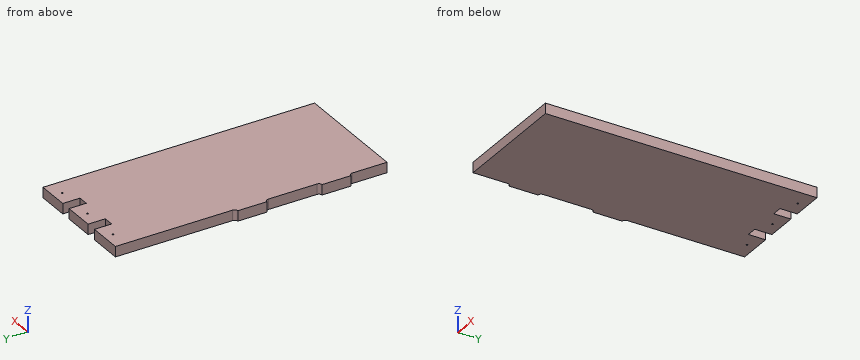
```python
from build123d import *

# Parameters (mm, degrees)
ESQUISSE1_R             = 0.127
ESQUISSE1_R_2           = 0.3999992
ESQUISSE1_R_3           = 0.4953
BOSS_EXTRU_1_DEPTH      = 1.55632912
ESQUISSE2_W             = 12.774737624
ESQUISSE2_H             = 41
ENL_V_MAT_EXTRU_1_DEPTH = 52.423945398


with BuildPart() as part:
    # Esquisse1 → Boss.-Extru.1 (new body)
    with BuildSketch(Plane(origin=(0, 0, 0), x_dir=(-1, 0, 0), z_dir=(0, 0, -1))):
        with BuildLine():
            Line((-12.23900032, 5.25), (-12.23900032, 0))
            Line((-12.23900032, 0), (0, 0))
            Line((0, 0), (0, 41))
            Line((0, 41), (-12.23900032, 41))
            Line((-12.23900032, 41), (-12.23900032, 23.299999237))
            ThreePointArc((-12.23900032, 23.299999237), (-12.74450016, 22.794499397), (-13.25, 23.299999237))
            Line((-13.25, 23.299999237), (-13.25, 41))
            Line((-13.25, 41), (-18.3939991, 41))
            Line((-18.3939991, 41), (-18.3939991, 38.400001526))
            Line((-18.3939991, 38.400001526), (-19.950000763, 38.400001526))
            Line((-19.950000763, 38.400001526), (-19.950000763, 41))
            Line((-19.950000763, 41), (-24.607000351, 41))
            Line((-24.607000351, 41), (-24.607000351, 38.400001526))
            Line((-24.607000351, 38.400001526), (-26.149999619, 38.400001526))
            Line((-26.149999619, 38.400001526), (-26.149999619, 41))
            Line((-26.149999619, 41), (-31, 41))
            Line((-31, 41), (-31, 0))
            Line((-31, 0), (-13.25, 0))
            Line((-13.25, 0), (-13.25, 5.25))
            ThreePointArc((-13.25, 5.25), (-12.74450016, 5.756000289), (-12.23900032, 5.25))
        make_face()
        with Locations(Location((-22.24999868, 39.64999944, 0), (0, 0, 180))):
            Circle(ESQUISSE1_R, mode=Mode.SUBTRACT)
        with Locations(Location((-28.44999898, 39.64999944, 0), (0, 0, 180))):
            Circle(ESQUISSE1_R, mode=Mode.SUBTRACT)
        with Locations(Location((-16.04999838, 39.64999944, 0), (0, 0, 180))):
            Circle(ESQUISSE1_R, mode=Mode.SUBTRACT)
        with Locations(Location((-8.7900002, 35.81500076, 0), (0, 0, 180))):
            Circle(ESQUISSE1_R_2, mode=Mode.SUBTRACT)
        with Locations(Location((-6.2500002, 38.35500076, 0), (0, 0, 180))):
            Circle(ESQUISSE1_R_2, mode=Mode.SUBTRACT)
        with Locations(Location((-3.7100002, 35.81500076, 0), (0, 0, 180))):
            Circle(ESQUISSE1_R_2, mode=Mode.SUBTRACT)
        with Locations(Location((-3.59000044, 6.14000042, 0), (0, 0, 180))):
            Circle(ESQUISSE1_R_3, mode=Mode.SUBTRACT)
        with Locations(Location((-1.05000044, 6.14000042, 0), (0, 0, 180))):
            Circle(ESQUISSE1_R_3, mode=Mode.SUBTRACT)
        with Locations(Location((-1.05000044, 1.06000042, 0), (0, 0, 180))):
            Circle(ESQUISSE1_R_3, mode=Mode.SUBTRACT)
        with Locations(Location((-1.05000044, 3.60000042, 0), (0, 0, 180))):
            Circle(ESQUISSE1_R_3, mode=Mode.SUBTRACT)
        with BuildLine():
            Line((-12.250000009, 17.899931304), (-12.251000404, 10.578000069))
            ThreePointArc((-12.251000404, 10.578000069), (-12.761750957, 10.078121146), (-13.25, 10.600000381))
            Line((-13.25, 10.600000381), (-13.25, 17.899999619))
            ThreePointArc((-13.25, 17.899999619), (-12.749965845, 18.399999615), (-12.250000009, 17.899931304))
        make_face(mode=Mode.SUBTRACT)
    extrude(amount=-BOSS_EXTRU_1_DEPTH)

    # Esquisse2 → Enlèv. mat.-Extru.1 (cut, through all)
    with BuildSketch(Plane.XY.offset(1.55632912)):
        with Locations((6.387368812, 20.5)):
            Rectangle(ESQUISSE2_W, ESQUISSE2_H)
    extrude(amount=-ENL_V_MAT_EXTRU_1_DEPTH, mode=Mode.SUBTRACT)


solid = part.part
```
Could you check a few things on this model? Use its own coordinates, in mm. Round coordinates to 2 decimals unless told otherwise and drop trailing zeros. Loops run counter-clockwise (first coordinate to the right, second up) from the corner with the lowest first, then second, coordinate; pieces in that order, holes last. Notation, with made-up numbers: (42.25, -12.75) - (92.25, -12.75) arc R27 cw to (92.25, 23.25) - close; hole circle Ø2 at (13.25, -24). An arc over 180 degrees is marked (long way). Answer as CSV lines item,"result".
1. For pin 1 Ø0.8 at (y, z) = (40, 1) entering from -X; pin 2 Ø0.5 at (x, z) = (25, 0.5) entering from +Y, each with a flat end and sliding along its axis, tell me the tip position at first contact or that it passes through.
Filled in:
pin 1,"stops at x = 13.25"
pin 2,"stops at y = 38.4"
2. Please list where these lines run through material, in increasing order: line 1 along X through (y, z) = (39.65, 1); line 2 along Y through (x, z) = (28.5, 1.1); line 3 along Y through (x, z) = (25.25, 0.3). Write a range as [from, to].
Filled in:
line 1,"x = [13.25, 15.92], [16.18, 18.39], [19.95, 22.12], [22.38, 24.61], [26.15, 28.32], [28.58, 31]"
line 2,"y = [0, 39.53], [39.77, 41]"
line 3,"y = [0, 38.4]"
3. I want a section at B-B on y = 14. List the corners of the cut face in (x, z) for me, then the cut area to 3 significant figures.
Filled in:
outline,"(13.25, 0) - (31, 0) - (31, 1.56) - (13.25, 1.56) - close"
area,"27.6 mm^2"
4. I want a section at A-A on z = 1.25. List the corners of the cut face in (x, y) for me.
Filled in:
outline,"(12.77, 5.76) arc R0.51 cw to (13.25, 5.25) - (13.25, 0) - (31, 0) - (31, 41) - (26.15, 41) - (26.15, 38.4) - (24.61, 38.4) - (24.61, 41) - (19.95, 41) - (19.95, 38.4) - (18.39, 38.4) - (18.39, 41) - (13.25, 41) - (13.25, 23.3) arc R0.51 cw to (12.77, 22.8) - (12.77, 18.4) arc R0.5 cw to (13.25, 17.9) - (13.25, 10.6) arc R0.5 cw to (12.77, 10.08) - close; hole circle Ø0.25 at (16.05, 39.65); hole circle Ø0.25 at (22.25, 39.65); hole circle Ø0.25 at (28.45, 39.65)"
